Source: CAD feature listing. Evaluate the final solid. Frame: model axes, mm. A direction names the side the tool comes from. Round coordinates to 2 decimals unless told otherwise and drop trailing zeros. Order: outer loops, then holes, each group sorted by start corner. A loop starts at its lowest first (then second) coordinate and runs counter-clockwise, first axis right, second up. Notation, with made-up numbers: (-38, 3.25) -> (-28, 3.25) arc R27 cw to (-28, 22.25) -> close; hole circle Ø4 at (-34, 10.25). An arc over 180 degrees is marked (long way). One line per item, written item: value. Start each with the question number.
1) Section D-D (y = 3.5). State how many separate pieces and enclosed holes the cut face has, and give its area (3 significant figures).
2) Section B-B (z = 20). Return the cut outline in (x, y).
3) Section C-C (z = 40). Return the cut outline in (x, y).
4) Mould query, pull axis Z, two halves, no side actions, for faces 6 (the face through (-26, 8, 36.5)), 7 (the face through (43.273, 2.958, -12.457)), 8 (the face through (-39, 8, 9)). Classes: pulls with the +Z half, pulls with the -Z half, needs draft (parallel to the pull), parting line crosses it, or undercut.
5) Section A-A (x = -21). Return the cut outline in (y, z), and give its area (3 significant figures).
6) Reachability of faces 1 (the face through (-31, 1, -17)), 2 (the face through (-26, 8, -20)), 3 (the face through (-13, 8, 9)), 4 (the face through (-26, 6, 28.5)), 5 (the face through (31.78, -0.99, -10.29)) from +Z, -Z, +X, -X, +Y, -Y: full face, straight path, thin tool, end or side. Return the list, or none.
7) Pin query (flat end, axial travel): P1, Ø6, axis at x = -7.5, z = 11, coming from the -Y side; P2, Ø2.5, axis at y = 8.5, z = 6, coming from the -X side; P3, Ø5, axis at x = -3.5, z = 35, coming from the +Y side. Return the tip coordinate at first contact, or that it passes through.
8) Ray query, L1, parallel to X at y = 1.4, z = -2.75; L2, parallel to X at y = 4.35, z = -12.75; L3, parallel to X at y = 4.25, z = 7. Return the intervals inside material, ascending.
```python
from build123d import *

# Parameters (mm, degrees)
SKETCH1_W           = 90
SKETCH1_H           = 90
BOSS_EXTRUDE1_DEPTH = 6
SKETCH2_W           = 26
SKETCH2_H           = 56.5
BOSS_EXTRUDE2_DEPTH = 5
SKETCH3_W           = 21
SKETCH3_H           = 40.5
CUT_EXTRUDE1_DEPTH  = 12
SKETCH4_R           = 2.25
CUT_EXTRUDE2_DEPTH  = 10
SKETCH5_R           = 1.75
CUT_EXTRUDE3_DEPTH  = 11
FILLET1_R           = 10
FILLET2_R           = 10
SKETCH6_R           = 2.25
CUT_EXTRUDE4_DEPTH  = 11
SKETCH7_R           = 9.5
SKETCH7_R_2         = 7.5
BOSS_EXTRUDE3_DEPTH = 2
SKETCH8_R           = 2.25
CUT_EXTRUDE5_DEPTH  = 10


with BuildPart() as part:
    # Sketch1 → Boss-Extrude1 (new body)
    with BuildSketch(Plane(origin=(0, 0, 0), x_dir=(1, 0, 0), z_dir=(0, 1, 0))):
        with Locations((0, -5)):
            Rectangle(SKETCH1_W, SKETCH1_H)
    extrude(amount=BOSS_EXTRUDE1_DEPTH)

    # Sketch2 → Boss-Extrude2 (add)
    with BuildSketch(Plane(origin=(0, 6, 0), x_dir=(1, 0, 0), z_dir=(0, 1, 0))):
        with Locations((-26, -8.25)):
            Rectangle(SKETCH2_W, SKETCH2_H)
    extrude(amount=BOSS_EXTRUDE2_DEPTH)

    # Sketch3 → Cut-Extrude1 (cut)
    with BuildSketch(Plane(origin=(0, 11, 0), x_dir=(1, 0, 0), z_dir=(0, 1, 0))):
        with Locations((-26, -8.25)):
            Rectangle(SKETCH3_W, SKETCH3_H)
    extrude(amount=-CUT_EXTRUDE1_DEPTH, mode=Mode.SUBTRACT)

    # Sketch4 → Cut-Extrude2 (cut)
    with BuildSketch(Plane(origin=(0, 11, 0), x_dir=(1, 0, 0), z_dir=(0, 1, 0))):
        with Locations(Location((-31, 16.5, 0), (0, 0, 270))):
            Circle(SKETCH4_R)
        with Locations(Location((-21, 16.5, 0), (0, 0, 270))):
            Circle(SKETCH4_R)
        with Locations(Location((-31, -33, 0), (0, 0, 270))):
            Circle(SKETCH4_R)
        with Locations(Location((-21, -33, 0), (0, 0, 270))):
            Circle(SKETCH4_R)
    extrude(amount=-CUT_EXTRUDE2_DEPTH, mode=Mode.SUBTRACT)

    # Sketch5 → Cut-Extrude3 (cut)
    with BuildSketch(Plane(origin=(0, 6, 0), x_dir=(1, 0, 0), z_dir=(0, 1, 0))):
        with Locations(Location((26, 2.75, 0), (0, 0, 270))):
            Circle(SKETCH5_R)
    extrude(amount=-CUT_EXTRUDE3_DEPTH, mode=Mode.SUBTRACT)

    # Fillet1
    fillet1_edges = [part.edges().sort_by_distance(p)[0] for p in [
        (-45, 3, -40),
    ]]
    fillet(fillet1_edges, radius=FILLET1_R)

    # Fillet2
    fillet2_edges = [part.edges().sort_by_distance(p)[0] for p in [
        (45, 3, -40),
    ]]
    fillet(fillet2_edges, radius=FILLET2_R)

    # Sketch6 → Cut-Extrude4 (cut)
    with BuildSketch(Plane(origin=(0, 0, 0), x_dir=(-1, 0, 0), z_dir=(0, -1, 0))):
        with Locations(Location((-41.042034918, 12.75, 0), (0, 0, 90))):
            Circle(SKETCH6_R)
        with Locations(Location((41.697396753, 12.75, 0), (0, 0, 90))):
            Circle(SKETCH6_R)
        with Locations(Location((-41.042034918, -7.25, 0), (0, 0, 90))):
            Circle(SKETCH6_R)
        with Locations(Location((41.697396753, -7.25, 0), (0, 0, 90))):
            Circle(SKETCH6_R)
    extrude(amount=-CUT_EXTRUDE4_DEPTH, mode=Mode.SUBTRACT)

    # Sketch7 → Boss-Extrude3 (add)
    with BuildSketch(Plane(origin=(0, 0, 0), x_dir=(-1, 0, 0), z_dir=(0, -1, 0))):
        with Locations(Location((-26, 2.75, 0), (0, 0, 270))):
            Circle(SKETCH7_R)
        with Locations(Location((-26, 2.75, 0), (0, 0, 90))):
            Circle(SKETCH7_R_2, mode=Mode.SUBTRACT)
    extrude(amount=BOSS_EXTRUDE3_DEPTH)

    # Sketch8 → Cut-Extrude5 (cut)
    with BuildSketch(Plane(origin=(0, 6, 0), x_dir=(1, 0, 0), z_dir=(0, 1, 0))):
        with Locations(Location((0, 0, 0), (0, 0, 270))):
            Circle(SKETCH8_R)
        with Locations(Location((0, -20, 0), (0, 0, 270))):
            Circle(SKETCH8_R)
        with Locations(Location((0, -40, 0), (0, 0, 270))):
            Circle(SKETCH8_R)
    extrude(amount=-CUT_EXTRUDE5_DEPTH, mode=Mode.SUBTRACT)


solid = part.part
```
Findings:
1. separate pieces: 1
1. enclosed holes: 13
1. area: 7,020 mm2
2. outline: (-45, 0) -> (-36.5, 0) -> (-36.5, 11) -> (-39, 11) -> (-39, 6) -> (-45, 6) -> close; (-15.5, 0) -> (-2.25, 0) -> (-2.25, 6) -> (-13, 6) -> (-13, 11) -> (-15.5, 11) -> close; (2.25, 0) -> (45, 0) -> (45, 6) -> (2.25, 6) -> close
3. outline: (-45, 0) -> (-2.25, 0) -> (-2.25, 6) -> (-45, 6) -> close; (2.25, 0) -> (45, 0) -> (45, 6) -> (2.25, 6) -> close
4. face 6: pulls with the +Z half
4. face 7: undercut
4. face 8: needs draft
5. outline: (0, -40) -> (6, -40) -> (6, -20) -> (11, -20) -> (11, -18.75) -> (1, -18.75) -> (1, -14.25) -> (11, -14.25) -> (11, -12) -> (0, -12) -> close; (0, 28.5) -> (11, 28.5) -> (11, 30.75) -> (1, 30.75) -> (1, 35.25) -> (11, 35.25) -> (11, 36.5) -> (6, 36.5) -> (6, 50) -> (0, 50) -> close
5. area: 287 mm2
6. face 1: +Y
6. face 2: -Z, +X, -X, +Y
6. face 3: +Z, -Z, +X, +Y
6. face 4: +Y, -Y
6. face 5: -Y
7. P1: y = 0
7. P2: x = -39
7. P3: y = 6
8. L1: -45 to -36.5, -15.5 to 24.25, 27.75 to 45
8. L2: -45 to -43.95, -39.45 to 38.79, 43.29 to 45
8. L3: -45 to -43.93, -39.46 to -36.5, -15.5 to 38.81, 43.28 to 45
